Build history of the part. All positions in model axes, mm. Face numbers are marked on the shaded views. A direction names the side the tool comes from. Round coordinates to 2 decimals unless told otherwise and drop trailing zeros. Write each loop counter-clockwise with the first axis right and the second up, starting at its lowest first coordinate (ties: lowest second). Pieces come first, ordered by that corner, then holes. Notation, with made-up numbers: (34, -40) -> (48, -40) arc R12 cw to (48, -30) -> close; hole circle Ø9 at (-24, 84). An arc over 180 degrees is marked (long way). Answer in a Markdown table with one row per item.
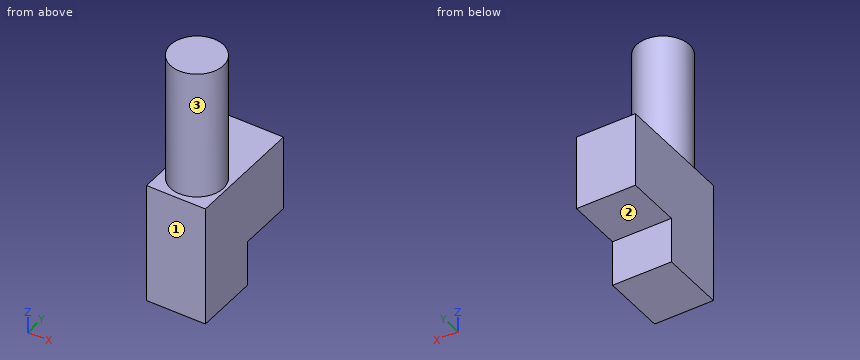
```python
from build123d import *

# Parameters (mm, degrees)
SKETCH1_W           = 29
SKETCH1_H           = 31.5
BOSS_EXTRUDE1_DEPTH = 59.5
BOSS_EXTRUDE2_START = 15.75
SKETCH2_W           = 29
SKETCH2_H           = 37
BOSS_EXTRUDE2_DEPTH = 27
BOSS_EXTRUDE3_START = 59.5
SKETCH4_R           = 13
BOSS_EXTRUDE3_DEPTH = 63.5


with BuildPart() as part:
    # Sketch1 → Boss-Extrude1 (new body)
    with BuildSketch(Plane.XY):
        Rectangle(SKETCH1_W, SKETCH1_H)
    extrude(amount=BOSS_EXTRUDE1_DEPTH)

    # Sketch2 → Boss-Extrude2 (add)
    with BuildSketch(Plane(origin=(0, 0, 0), x_dir=(1, 0, 0), z_dir=(0, 1, 0)).offset(BOSS_EXTRUDE2_START)):
        with Locations((0, -41)):
            Rectangle(SKETCH2_W, SKETCH2_H)
    extrude(amount=BOSS_EXTRUDE2_DEPTH)

    # Sketch4 → Boss-Extrude3 (add)
    with BuildSketch(Plane.XY.offset(BOSS_EXTRUDE3_START)):
        with Locations(Location((0, 0, 0), (0, 0, 180))):
            Circle(SKETCH4_R)
    extrude(amount=BOSS_EXTRUDE3_DEPTH)


solid = part.part
```
Q1. Wall check: line 1 (Z direction, x = 5.5, y = 15.5); line 2 (Y direction, x = 0, z = 78); line 3 (Z direction, x = 8.75, y = 27). Give the ranges that are in metal, low to high. Write a range as [from, to].
A:
| item | result |
|---|---|
| line 1 | [0, 59.5] |
| line 2 | [-13, 13] |
| line 3 | [22.5, 59.5] |
Q2. Drop flat-ended pins along their axis: P1, Ø8, axis at x = 6, y = 30, coming from the -Z side; P2, Ø4, axis at x = 1, z = 96.5, coming from the -Y side; P3, Ø1, axis at x = 1.5, y = 16.5, coming from the +Z side. Give the stop position or say it passes through.
A:
| item | result |
|---|---|
| P1 | z = 22.5 |
| P2 | y = -13 |
| P3 | z = 59.5 |
Q3. Which spindle directions (+Z, -Z, +X, -X, +Y, -Y) get a long thin tool onto all of the face, cutting with end or side? Do the marked faces 1, 2 and 3. Say none if no direction does.
A:
| item | result |
|---|---|
| face 1 | +Z, -Z, +X, -X, -Y |
| face 2 | -Z, +X, -X, +Y |
| face 3 | +Z |
Q4. Saw through at B-B on y = 0. Write the cut outline in (x, z), plus the area to 3 significant figures.
A:
| item | result |
|---|---|
| outline | (-14.5, 0) -> (14.5, 0) -> (14.5, 59.5) -> (13, 59.5) -> (13, 123) -> (-13, 123) -> (-13, 59.5) -> (-14.5, 59.5) -> close |
| area | 3,380 mm² |
Q5. Saw through at A-A on x = 0. Write the cut outline in (y, z).
A:
| item | result |
|---|---|
| outline | (-15.75, 0) -> (15.75, 0) -> (15.75, 22.5) -> (42.75, 22.5) -> (42.75, 59.5) -> (13, 59.5) -> (13, 123) -> (-13, 123) -> (-13, 59.5) -> (-15.75, 59.5) -> close |
Q6. Saw through at D-D on x = -10.75. Write the cut outline in (y, z).
A:
| item | result |
|---|---|
| outline | (-15.75, 0) -> (15.75, 0) -> (15.75, 22.5) -> (42.75, 22.5) -> (42.75, 59.5) -> (7.31, 59.5) -> (7.31, 123) -> (-7.31, 123) -> (-7.31, 59.5) -> (-15.75, 59.5) -> close |
Q7. Saw through at C-C on z = 61. Write the cut outline in (x, y).
A:
| item | result |
|---|---|
| outline | circle Ø26 at (0, 0) |
